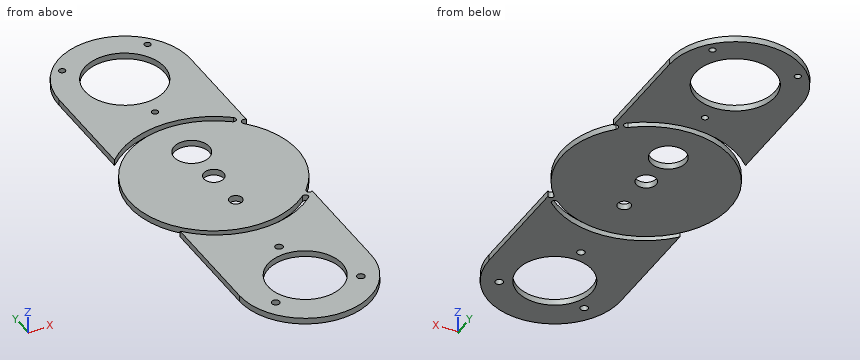
from build123d import *

# Parameters (mm, degrees)
SKETCH003_R                = 54.85
SKETCH003_R_2              = 11.5
SKETCH003_R_3              = 6.5
SKETCH003_R_4              = 4.25
EXTRUDE010_DEPTH           = 4
EXTRUDE011_DEPTH           = 4
SKETCH_R                   = 24.25
SKETCH_R_2                 = 2.5
EXTRUDE008_DEPTH           = 4
SKETCH001_R                = 26
SKETCH001_R_2              = 2.1
EXTRUDE007_DEPTH           = 4
EXTRUDE007_PLACEMENT_ANGLE = 180


with BuildPart() as cap001:
    # Sketch003 (on Face2 of Tube) → Extrude010 (new body)
    with BuildSketch(Plane.XY.offset(150)):
        Circle(SKETCH003_R)
        with Locations((0, 27)):
            Circle(SKETCH003_R_2, mode=Mode.SUBTRACT)
        Circle(SKETCH003_R_3, mode=Mode.SUBTRACT)
        with Locations((0, -27)):
            Circle(SKETCH003_R_4, mode=Mode.SUBTRACT)
    extrude(amount=EXTRUDE010_DEPTH)


with BuildPart() as cap001_1:
    # Extrude010 placement: moved
    add(cap001.part.moved(Location((190, 0, -150))))


with BuildPart() as fusion:
    # Sketch005 → Extrude011 (new body)
    with BuildSketch(Plane.XY):
        with BuildLine():
            ThreePointArc((233, 40.844952), (229.858715, 40.897579), (229.786368, 37.756687))
            ThreePointArc((229.786368, 37.756687), (227.249454, 40.261653), (224.555163, 42.596517))
            ThreePointArc((224.555163, 42.596517), (227.636022, 42.926115), (227.289643, 46.005133))
            ThreePointArc((233, 40.844952), (230.227647, 43.516698), (227.289643, 46.005133))
        make_face()
        with BuildLine():
            ThreePointArc((230.295506, -37.21283), (230.41557, -39.799082), (233, -39.644688))
            ThreePointArc((228.114531, -44.584093), (230.632391, -42.188696), (233, -39.644688))
            ThreePointArc((228.114531, -44.584093), (228.278175, -41.913762), (225.609951, -41.718748))
            ThreePointArc((225.609951, -41.718748), (228.01954, -39.535264), (230.295506, -37.21283))
        make_face()
    extrude(amount=EXTRUDE011_DEPTH)

    # Fusion: union Cap001
    add(cap001_1.part)


with BuildPart() as fusion001:
    # Sketch → Extrude008 (new body)
    with BuildSketch(Plane.XY):
        with BuildLine():
            ThreePointArc((-43, -37.644688), (0, -57.15), (43, -37.644688))
            Line((43, -37.644688), (43, -110))
            ThreePointArc((-43, -110), (0, -153), (43, -110))
            Line((-43, -37.644688), (-43, -110))
        make_face()
        with Locations((0, -110)):
            Circle(SKETCH_R, mode=Mode.SUBTRACT)
        with Locations((0, -77.95706)):
            Circle(SKETCH_R_2, mode=Mode.SUBTRACT)
        with Locations((-27.75, -126.02147)):
            Circle(SKETCH_R_2, mode=Mode.SUBTRACT)
        with Locations((27.75, -126.02147)):
            Circle(SKETCH_R_2, mode=Mode.SUBTRACT)
    extrude(amount=EXTRUDE008_DEPTH)


with BuildPart() as fusion001_1:
    # Extrude008 placement: moved
    add(fusion001.part.moved(Location((190, -2, 0))))

    # Fusion001: union Fusion
    add(fusion.part)


with BuildPart() as fusion002:
    # Sketch001 → Extrude007 (new body)
    with BuildSketch(Plane.XY):
        with BuildLine():
            ThreePointArc((-43, -41.844952), (0, -60), (43, -41.844952))
            Line((43, -41.844952), (43, -110))
            ThreePointArc((-43, -110), (0, -153), (43, -110))
            Line((-43, -41.844952), (-43, -110))
        make_face()
        with Locations((0, -110)):
            Circle(SKETCH001_R, mode=Mode.SUBTRACT)
        with Locations((0, -72.942541)):
            Circle(SKETCH001_R_2, mode=Mode.SUBTRACT)
        with Locations((27.875, -134.418019)):
            Circle(SKETCH001_R_2, mode=Mode.SUBTRACT)
        with Locations((-27.875, -134.418019)):
            Circle(SKETCH001_R_2, mode=Mode.SUBTRACT)
    extrude(amount=EXTRUDE007_DEPTH)


with BuildPart() as fusion002_1:
    # Extrude007 placement: moved
    add(fusion002.part.moved(Location((190, -1, 0))).rotate(Axis((190, -1, 0), (0, 0, 1)), EXTRUDE007_PLACEMENT_ANGLE))

    # Fusion002: union Fusion001
    add(fusion001_1.part)


solid = fusion002_1.part
Read the model definition and answer for the solid it produces. Units are mm, in the model's axes. Coordinates: 2 decimals unless noted, no trailing zeros. Loops run counter-clockwise (first coordinate to the right, second up) from the corner with the lowest first, then second, coordinate; pieces in that order, holes last.
Q1. The part is cut by section B-B on z = 1.1. Give the number of separate pieces and of enclosed holes in the cut face, and give its area (3 significant figures).
Q2. The part is cut by section A-A on y = 0. Write down the section's boundary in (x, z), and give its area (3 significant figures).
Q3. Each of these flat-tipped pins is pushed along its axis until it touches: pin 1 Ø1.5 at (x, z) = (183.5, 2) entering from -Y; pin 2 Ø1.2 at (y, z) = (-93.5, 3) entering from -X; pin 3 Ø1 at (y, z) = (-91.5, 1.5) entering from +X. Where does it stop, or does it pass through?
Q4. Consider probe 1 along Y at (x, z) = (220.5, 1.5); probe 2 along Y at (x, z) = (162.25, 1.45); probe 3 along X at (y, z) = (42.5, 1.15). Determine where each line is inside the solid, lowest interval first.
Q5. The part is cut by section C-C on y = 87. Write down the section's boundary in (x, z), and give its area (3 significant figures).
Q6. The part is cut by section D-D on x = 237. Write down the section's boundary in (y, z), and give its area (3 significant figures).
Results below:
1. separate pieces: 1
1. enclosed holes: 11
1. area: 20,500 mm2
2. outline: (135.15, 0) - (183.5, 0) - (183.5, 4) - (135.15, 4) - close; (196.5, 0) - (244.85, 0) - (244.85, 4) - (196.5, 4) - close
2. area: 387 mm2
3. pin 1: stops at y = -154.61
3. pin 2: stops at x = 147
3. pin 3: stops at x = 233
4. probe 1: y = -142.31 to -50.33, -45.59 to 45.59, 50.67 to 139.31
4. probe 2: y = -144.85 to -130.52, -125.52 to -51.96, -47.31 to 47.31, 52.2 to 131.32, 135.51 to 141.85
4. probe 3: x = 147 to 148.68, 155.33 to 224.68, 227.18 to 233
5. outline: (147, 0) - (176.14, 0) - (176.14, 4) - (147, 4) - close; (203.86, 0) - (233, 0) - (233, 4) - (203.86, 4) - close
5. area: 233 mm2
6. outline: (-28.28, 0) - (28.28, 0) - (28.28, 4) - (-28.28, 4) - close
6. area: 226 mm2
